Work out the finished part from the listing and answer in its coordinate system (mm). Face numbers are marked on the shaded views. A direction names the side the tool comes from. Coordinates: 2 decimals unless noted, no trailing zeros. Write each loop counter-clockwise with the first axis right and the second up, starting at its lowest first coordinate (ties: lowest second). Pieces come first, ordered by that corner, then holes. Notation, with made-up numbers: (13.5, 58) - (26.5, 58) arc R21 cw to (26.5, 84) - close; hole circle Ø11 at (40, -11). An arc over 180 degrees is marked (long way). One line per item, written item: value.
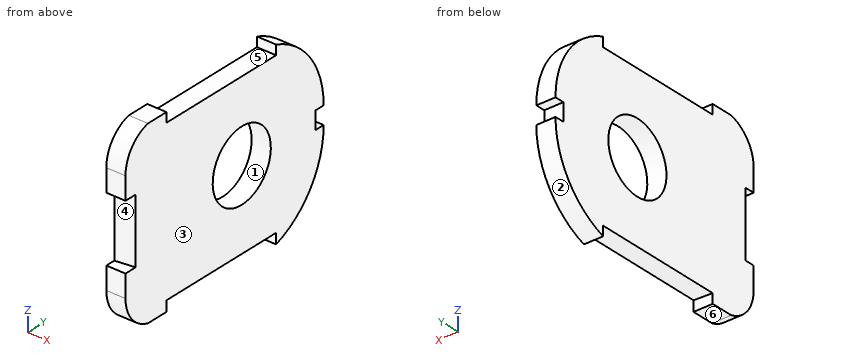
```python
from build123d import *

# Parameters (mm, degrees)
SKETCH1_R           = 11
BOSS_EXTRUDE1_DEPTH = 6
CUT_EXTRUDE3_DEPTH  = 41.5
CUT_EXTRUDE5_DEPTH  = 20.4


with BuildPart() as part:
    # Sketch1 → Boss-Extrude1 (new body)
    with BuildSketch(Plane(origin=(0, 0, 0), x_dir=(0, 0, -1), z_dir=(1, 0, 0))):
        with BuildLine():
            Line((-10.2, -3), (-10.2, 0))
            Line((-10.2, 0), (10.2, 0))
            Line((10.2, 0), (10.2, -3))
            Line((10.2, -3), (17.2, -3))
            ThreePointArc((17.2, -3), (24.071862921, -0.620131711), (28, 5.5))
            Line((28, 5.5), (28, 12.5))
            Line((28, 12.5), (25, 12.5))
            Line((25, 12.5), (25, 41))
            Line((25, 41), (25, 54))
            Line((25, 54), (28, 54))
            ThreePointArc((28, 54), (18.254535627, 67.039348587), (2.75, 72))
            Line((2.75, 72), (2.75, 69))
            Line((2.75, 69), (-2.75, 69))
            Line((-2.75, 69), (-2.75, 72))
            ThreePointArc((-2.75, 72), (-18.254535627, 67.039348587), (-28, 54))
            Line((-28, 54), (-25, 54))
            Line((-25, 54), (-25, 41))
            Line((-25, 41), (-25, 12.5))
            Line((-25, 12.5), (-28, 12.5))
            Line((-28, 12.5), (-28, 5.5))
            ThreePointArc((-28, 5.5), (-24.071862921, -0.620131711), (-17.2, -3))
            Line((-17.2, -3), (-10.2, -3))
        make_face()
        with Locations((0, 41)):
            Circle(SKETCH1_R, mode=Mode.SUBTRACT)
    extrude(amount=BOSS_EXTRUDE1_DEPTH)

    # Sketch5 → Cut-Extrude3 (cut)
    with BuildSketch(Plane.XZ.offset(-54)):
        Polygon((0, -25), (6, -25), (6, -24.751672534), align=None)
    extrude(amount=CUT_EXTRUDE3_DEPTH, mode=Mode.SUBTRACT)

    # Sketch6 → Cut-Extrude5 (cut)
    with BuildSketch(Plane.XY.offset(-10.2)):
        Polygon((0, 0), (6, 0), (6, 0.843245008), align=None)
    extrude(amount=CUT_EXTRUDE5_DEPTH, mode=Mode.SUBTRACT)


solid = part.part
```
Item 1: Section B-B, the plane y = 41 is taken. Determine the outline of the cut face in (x, z).
Evaluation:
outline: (0, -25) - (6, -24.75) - (6, -11) - (0, -11) - close; (0, 11) - (6, 11) - (6, 25) - (0, 25) - close
Item 2: Section D-D, the plane y = 19 is taken. Determine the outline of the cut face in (x, z), then the cut area to 3 significant figures.
Evaluation:
outline: (0, -25) - (6, -24.75) - (6, 25) - (0, 25) - close
area: 299 mm2
Item 3: Section C-C, the plane x = 1.5 is taken. Determine the outline of the cut face in (y, z).
Evaluation:
outline: (-3, -17.2) arc R11.11 ccw to (5.5, -28) - (12.5, -28) - (12.5, -24.94) - (54, -24.94) - (54, -28) arc R26.71 ccw to (72, -2.75) - (69, -2.75) - (69, 2.75) - (72, 2.75) arc R26.71 ccw to (54, 28) - (54, 25) - (12.5, 25) - (12.5, 28) - (5.5, 28) arc R11.11 ccw to (-3, 17.2) - (-3, 10.2) - (0.21, 10.2) - (0.21, -10.2) - (-3, -10.2) - close; hole circle Ø22 at (41, 0)
Item 4: Section A-A, the plane z = 0 is taken. Determine the outline of the cut face in (x, y).
Evaluation:
outline: (0, 0) - (6, 0.84) - (6, 30) - (0, 30) - close; (0, 52) - (6, 52) - (6, 69) - (0, 69) - close
Item 5: Consider probe 1 along Y at (x, z) = (0.75, 9); probe 2 along Y at (x, z) = (4.75, 0); probe 3 along Z at (x, y) = (3, 46). Determine where each line is inside the solid, lowest interval first.
Evaluation:
probe 1: y = 0.11 to 34.68, 47.32 to 71.26
probe 2: y = 0.67 to 30, 52 to 69
probe 3: z = -24.88 to -9.8, 9.8 to 25
Item 6: Given pin 1 (2.5 mm diameter, centred on x = 3.5, z = 26, fed in from +Y); pin 2 (1.6 mm diameter, centred on x = 3.5, z = -26, fed in from -Y); pin 3 (6 mm diameter, centred on y = 50.5, z = 5.5, fed in from -X); pin 4 (3 mm diameter, centred on x = 2, y = -1.5, fed in from +Z), each flat-ended and moving along its own axis, determine where each tip first touches the part or whether it passes through.
Evaluation:
pin 1: stops at y = 60.44
pin 2: stops at y = 0.4
pin 3: stops at x = 0
pin 4: stops at z = 24.79
Item 7: Determine the mould class of the marked faces 1, 2 and 3 for opening direction Y: +Y half, -Y half, draft (parallel to the pull), parting line (faces both ways), or undercut.
Evaluation:
face 1: undercut
face 2: +Y half
face 3: draft
Item 8: Which of the six approach directions +Z, -Z, +X, -X, +Y, -Y give full straight-line access (tool end or side, diameter ignored) to the marked faces 4, 5 and 6?
Evaluation:
face 4: +X, -Y
face 5: +Z, +X, -X
face 6: -Z, +X, -X, +Y, -Y
